from build123d import *

# Parameters (mm, degrees)
P_IDAT_VYSUNUT_M1_DEPTH        = 5
SKICA5_W                       = 10.15
SKICA5_H                       = 360
P_IDAT_VYSUNUT_M5_DEPTH        = 7.15
ODEBRAT_VYSUNUT_M1_DEPTH       = 213.956673997
ODEBRAT_VYSUNUT_M1_DEPTH_BACK  = 213.956673997
SKICA9_R                       = 2
ODEBRAT_VYSUNUT_M3_DEPTH       = 213.956673997
SKICA13_R                      = 3.5
ODEBRAT_VYSUNUT_M9_DEPTH       = 9.15
P_IDAT_VYSUNUT_M6_DEPTH        = 5
SKICA15_R                      = 4
P_IDAT_VYSUNUT_M7_DEPTH        = 5
SKICA16_R                      = 2
ODEBRAT_VYSUNUT_M10_DEPTH      = 213.729981432
SKICA17_R                      = 3.5
ODEBRAT_VYSUNUT_M11_DEPTH      = 2
LINPOLE1_COUNT                 = 2
LINPOLE1_PITCH                 = 114
ODEBRAT_VYSUNUT_M12_DEPTH      = 378.430847971
ODEBRAT_VYSUNUT_M12_DEPTH_BACK = 378.430847971
SKICA18_W                      = 10.15
SKICA18_H                      = 2


with BuildPart() as part:
    # Skica1 → Přidat vysunutím1 (new body)
    with BuildSketch(Plane.XY):
        Polygon((113.15, -180), (113.15, 180), (103, 180), (103, 177), (-103, 177), (-103, 180), (-113.15, 180), (-113.15, -180), (-103, -180), (-103, -177), (103, -177), (103, -180), align=None)
    extrude(amount=P_IDAT_VYSUNUT_M1_DEPTH)

    # Skica5 → Přidat vysunutím5 (add)
    with BuildSketch(Plane(origin=(0, 0, 0), x_dir=(-1, 0, 0), z_dir=(0, 0, -1))):
        with Locations((108.075, 0)):
            Rectangle(SKICA5_W, SKICA5_H)
        with Locations((-108.075, 0)):
            Rectangle(SKICA5_W, SKICA5_H)
    extrude(amount=P_IDAT_VYSUNUT_M5_DEPTH)

    # Skica7 → Odebrat vysunutím1 (cut, two sides: drawn at the far end of the back side and taken through both)
    with BuildSketch(Plane.XY.offset(5).offset(-ODEBRAT_VYSUNUT_M1_DEPTH_BACK)):
        with BuildLine():
            Line((12, 167), (87, 167))
            ThreePointArc((87, 167), (92.303300859, 164.803300859), (94.5, 159.5))
            Line((94.5, 159.5), (94.5, 69.5))
            ThreePointArc((94.5, 69.5), (92.303300859, 64.196699141), (87, 62))
            Line((87, 62), (12, 62))
            ThreePointArc((12, 62), (6.696699141, 64.196699141), (4.5, 69.5))
            Line((4.5, 69.5), (4.5, 159.5))
            ThreePointArc((4.5, 159.5), (6.696699141, 164.803300859), (12, 167))
        make_face()
        with BuildLine():
            Line((-12, 167), (-87, 167))
            ThreePointArc((-87, 167), (-92.303300859, 164.803300859), (-94.5, 159.5))
            Line((-94.5, 159.5), (-94.5, 69.5))
            ThreePointArc((-94.5, 69.5), (-92.303300859, 64.196699141), (-87, 62))
            Line((-87, 62), (-12, 62))
            ThreePointArc((-12, 62), (-6.696699141, 64.196699141), (-4.5, 69.5))
            Line((-4.5, 69.5), (-4.5, 159.5))
            ThreePointArc((-4.5, 159.5), (-6.696699141, 164.803300859), (-12, 167))
        make_face()
        with BuildLine():
            Line((94.5, 45), (94.5, -45))
            ThreePointArc((94.5, -45), (92.303300859, -50.303300859), (87, -52.5))
            Line((87, -52.5), (12, -52.5))
            ThreePointArc((12, -52.5), (6.696699141, -50.303300859), (4.5, -45))
            Line((4.5, -45), (4.5, 45))
            ThreePointArc((4.5, 45), (6.696699141, 50.303300859), (12, 52.5))
            Line((12, 52.5), (87, 52.5))
            ThreePointArc((87, 52.5), (92.303300859, 50.303300859), (94.5, 45))
        make_face()
        with BuildLine():
            Line((-94.5, 45), (-94.5, -45))
            ThreePointArc((-94.5, -45), (-92.303300859, -50.303300859), (-87, -52.5))
            Line((-87, -52.5), (-12, -52.5))
            ThreePointArc((-12, -52.5), (-6.696699141, -50.303300859), (-4.5, -45))
            Line((-4.5, -45), (-4.5, 45))
            ThreePointArc((-4.5, 45), (-6.696699141, 50.303300859), (-12, 52.5))
            Line((-12, 52.5), (-87, 52.5))
            ThreePointArc((-87, 52.5), (-92.303300859, 50.303300859), (-94.5, 45))
        make_face()
        with BuildLine():
            Line((94.5, -69.5), (94.5, -159.5))
            ThreePointArc((94.5, -159.5), (92.303300859, -164.803300859), (87, -167))
            Line((87, -167), (12, -167))
            ThreePointArc((12, -167), (6.696699141, -164.803300859), (4.5, -159.5))
            Line((4.5, -159.5), (4.5, -69.5))
            ThreePointArc((4.5, -69.5), (6.696699141, -64.196699141), (12, -62))
            Line((12, -62), (87, -62))
            ThreePointArc((87, -62), (92.303300859, -64.196699141), (94.5, -69.5))
        make_face()
        with BuildLine():
            Line((-94.5, -69.5), (-94.5, -159.5))
            ThreePointArc((-94.5, -159.5), (-92.303300859, -164.803300859), (-87, -167))
            Line((-87, -167), (-12, -167))
            ThreePointArc((-12, -167), (-6.696699141, -164.803300859), (-4.5, -159.5))
            Line((-4.5, -159.5), (-4.5, -69.5))
            ThreePointArc((-4.5, -69.5), (-6.696699141, -64.196699141), (-12, -62))
            Line((-12, -62), (-87, -62))
            ThreePointArc((-87, -62), (-92.303300859, -64.196699141), (-94.5, -69.5))
        make_face()
    extrude(amount=ODEBRAT_VYSUNUT_M1_DEPTH + ODEBRAT_VYSUNUT_M1_DEPTH_BACK, mode=Mode.SUBTRACT)

    # Skica9 → Odebrat vysunutím3 (cut, through all)
    with BuildSketch(Plane(origin=(0, 0, -7.15), x_dir=(-1, 0, 0), z_dir=(0, 0, -1))):
        with Locations((98, 162)):
            Circle(SKICA9_R)
        with Locations((98, 54)):
            Circle(SKICA9_R)
        with Locations((98, -162)):
            Circle(SKICA9_R)
        with Locations((98, -60)):
            Circle(SKICA9_R)
    odebrat_vysunut_m3 = extrude(amount=-ODEBRAT_VYSUNUT_M3_DEPTH, mode=Mode.SUBTRACT)

    # Zrcadlit2: Odebrat vysunutím3 across plane
    add(odebrat_vysunut_m3.mirror(Plane(origin=(0, 0, 0), x_dir=(0, 0, 1), z_dir=(1, 0, 0))), mode=Mode.SUBTRACT)

    # Skica13 → Odebrat vysunutím9 (cut)
    with BuildSketch(Plane(origin=(0, 0, -7.15), x_dir=(-1, 0, 0), z_dir=(0, 0, -1))):
        with Locations((98, 162)):
            Circle(SKICA13_R)
        with Locations((98, 54)):
            Circle(SKICA13_R)
        with Locations((98, -162)):
            Circle(SKICA13_R)
        with Locations((98, -60)):
            Circle(SKICA13_R)
    odebrat_vysunut_m9 = extrude(amount=-ODEBRAT_VYSUNUT_M9_DEPTH, mode=Mode.SUBTRACT)

    # Zrcadlit3: Odebrat vysunutím9 across plane
    add(odebrat_vysunut_m9.mirror(Plane(origin=(0, 0, 0), x_dir=(0, 0, 1), z_dir=(1, 0, 0))), mode=Mode.SUBTRACT)

    # Skica14 → Přidat vysunutím6 (add)
    with BuildSketch(Plane(origin=(0, 0, 0), x_dir=(-1, 0, 0), z_dir=(0, 0, -1))):
        with BuildLine():
            Line((94.5, 71.5), (94.5, 41.5))
            ThreePointArc((94.5, 41.5), (92.303300859, 46.803300859), (87, 49))
            Line((87, 49), (12, 49))
            ThreePointArc((12, 49), (6.696699141, 46.803300859), (4.5, 41.5))
            Line((4.5, 41.5), (4.5, 71.5))
            ThreePointArc((4.5, 71.5), (6.696699141, 66.196699141), (12, 64))
            Line((12, 64), (87, 64))
            ThreePointArc((87, 64), (92.303300859, 66.196699141), (94.5, 71.5))
        make_face()
    p_idat_vysunut_m6 = extrude(amount=-P_IDAT_VYSUNUT_M6_DEPTH)

    # Skica15 → Přidat vysunutím7 (add)
    with BuildSketch(Plane(origin=(0, 0, 0), x_dir=(-1, 0, 0), z_dir=(0, 0, -1))):
        with BuildLine():
            Line((87, 15.5), (69.5, 15.5))
            ThreePointArc((69.5, 15.5), (64.196699141, 13.303300859), (62, 8))
            Line((62, 8), (62, -8))
            ThreePointArc((62, -8), (64.196699141, -13.303300859), (69.5, -15.5))
            Line((69.5, -15.5), (87, -15.5))
            ThreePointArc((87, -15.5), (92.303300859, -17.696699141), (94.5, -23))
            Line((94.5, -23), (94.5, 23))
            ThreePointArc((94.5, 23), (92.303300859, 17.696699141), (87, 15.5))
        make_face()
        with Locations((85.5, 6.5)):
            Circle(SKICA15_R, mode=Mode.SUBTRACT)
    extrude(amount=-P_IDAT_VYSUNUT_M7_DEPTH)

    # Skica16 → Odebrat vysunutím10 (cut, through all)
    with BuildSketch(Plane(origin=(0, 0, 0), x_dir=(-1, 0, 0), z_dir=(0, 0, -1))):
        with Locations((85.5, -11)):
            Circle(SKICA16_R)
    extrude(amount=-ODEBRAT_VYSUNUT_M10_DEPTH, mode=Mode.SUBTRACT)

    # Skica17 → Odebrat vysunutím11 (cut)
    with BuildSketch(Plane(origin=(0, 0, 0), x_dir=(-1, 0, 0), z_dir=(0, 0, -1))):
        with Locations((85.5, -11)):
            Circle(SKICA17_R)
    extrude(amount=-ODEBRAT_VYSUNUT_M11_DEPTH, mode=Mode.SUBTRACT)

    # LinPole1: Přidat vysunutím6 ×2
    with Locations(*[(0, -i * LINPOLE1_PITCH, 0) for i in range(1, LINPOLE1_COUNT)]):
        add(p_idat_vysunut_m6)

    # Skica18 → Odebrat vysunutím12 (cut, two sides: drawn at the far end of the back side and taken through both)
    with BuildSketch(Plane(origin=(0, 180, 0), x_dir=(1, 0, 0), z_dir=(0, 1, 0)).offset(-ODEBRAT_VYSUNUT_M12_DEPTH_BACK)):
        with Locations((-108.075, -4)):
            Rectangle(SKICA18_W, SKICA18_H)
        with Locations((108.075, -4)):
            Rectangle(SKICA18_W, SKICA18_H)
    extrude(amount=ODEBRAT_VYSUNUT_M12_DEPTH + ODEBRAT_VYSUNUT_M12_DEPTH_BACK, mode=Mode.SUBTRACT)


solid = part.part
For this review, take the finished solid that the model builds, in its own axes (mm). A direction names the side the tool comes from. Give positions to 0.01 mm unless a question says otherwise; leave off trailing zeros. Loops run counter-clockwise (first coordinate to the right, second up) from the corner with the lowest first, then second, coordinate; pieces in that order, holes last.
Item 1: For line 1 along X through (y, z) = (134, 1.5); line 2 along Y through (x, z) = (98, 0.6); line 3 along Y through (x, z) = (98, 2.65), list the stretches that pass through material, from the lowest coordinate up.
Item 2: Take a section at D-D, the plane x = 82. State the section outline as (y, z) points.
Item 3: Take a section at B-B, the plane x = -44. State the section outline as (y, z) points.
Item 4: Tool access review of faces 5 (the flat face through (0, 14, 0)), 6 (the flat face through (100, 160, 2)), 7 (the cylindrical face through (-92.245, -17.639, 2.465)): name each direction out of +Z, -Z, +X, -X, +Y, -Y from which nothing blocks a thin tool from reaching the whole face with its end or side.
Item 5: Take a section at A-A, the plane y = -145. State the section outline as (x, z) points.
Item 6: Insertion check: pin 1 (4.5 mm diameter, centred on x = -98, y = -162, fed in from -Z); pin 2 (5.5 mm diameter, centred on x = 47.5, z = 2.5, fed in from +Y); pin 3 (4 mm diameter, centred on x = 64, z = -1, fed in from -Y). Each pin has a flat end and moves straight along its axis. Give the tip position at first contact, or say it passes through.
Item 7: Draft analysis for pull direction X (two halves, no side actions). For faces 1 (the flat face through (108, -3, 3)), 2 (the flat face through (113.15, -3, -2)), 3 (the cylindrical face through (-92.361, -67.255, 2.465)), 4 (the cylindrical face through (-64.255, 13.361, 2.465)), state which applies: +X half, -X half, draft (parallel to the pull), parting line (faces both ways), or undercut.
Item 8: Take a section at C-C, the plane z = -4.25. State the section outline as (x, y) points, and give its area (3 significant figures).
Calculated:
1. line 1: x = -113.15 to -94.5, -4.5 to 4.5, 94.5 to 113.15
1. line 2: y = -177 to -165.5, -158.5 to -63.5, -56.5 to 50.5, 57.5 to 158.5, 165.5 to 177
1. line 3: y = -177 to -164, -160 to -62, -58 to 52, 56 to 160, 164 to 177
2. outline: (-177, 0) - (-167, 0) - (-167, 5) - (-177, 5) - close; (-62, 0) - (-52.5, 0) - (-52.5, 5) - (-62, 5) - close; (52.5, 0) - (62, 0) - (62, 5) - (52.5, 5) - close; (167, 0) - (177, 0) - (177, 5) - (167, 5) - close
3. outline: (-177, 0) - (-167, 0) - (-167, 5) - (-177, 5) - close; (-65, 0) - (-50, 0) - (-50, 5) - (-65, 5) - close; (49, 0) - (64, 0) - (64, 5) - (49, 5) - close; (167, 0) - (177, 0) - (177, 5) - (167, 5) - close
4. face 5: -Z, +Y, -Y
4. face 6: -Z
4. face 7: +Z, -Z
5. outline: (-113.15, -7.15) - (-103, -7.15) - (-103, 0) - (-94.5, 0) - (-94.5, 5) - (-103, 5) - (-103, 3) - (-113.15, 3) - close; (-4.5, 0) - (4.5, 0) - (4.5, 5) - (-4.5, 5) - close; (94.5, 0) - (103, 0) - (103, -7.15) - (113.15, -7.15) - (113.15, 3) - (103, 3) - (103, 5) - (94.5, 5) - close
6. pin 1: stops at z = 2
6. pin 2: stops at y = 177
6. pin 3: stops at y = -177
7. face 1: draft
7. face 2: +X half
7. face 3: undercut
7. face 4: undercut
8. outline: (-113.15, -180) - (-103, -180) - (-103, 180) - (-113.15, 180) - close; (103, -180) - (113.15, -180) - (113.15, 180) - (103, 180) - close
8. area: 7,310 mm2
